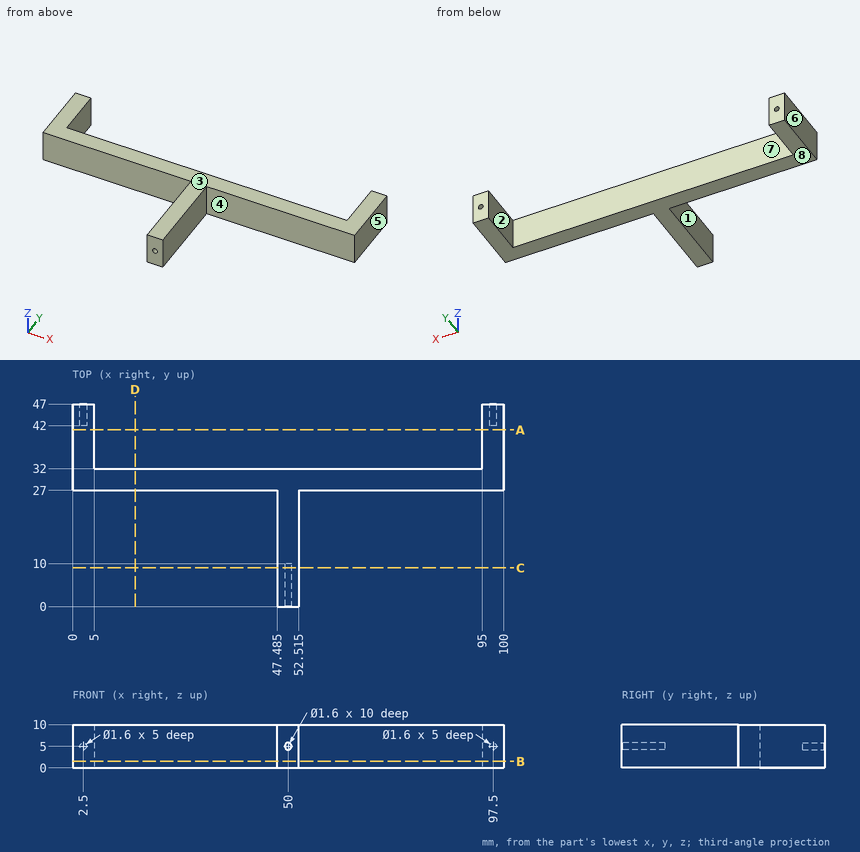
Check sheet for the drawn part. Datum: minimum x, y, z corner. Units: mm. A direction names the side the tool comes from. Give positions to 0.01 mm unless a question says otherwise; leave off trailing zeros. Write each loop counter-clockwise with the first axis right and the second up, starting at its lowest first coordinate (ties: lowest second). Pieces come first, ordered by that corner, then holes. Notation, with made-up numbers: M -34,26.25 L 25,26.25 A4 cw 25,32.25 Z; hole C 51,77.25 d3. An arc over 180 degrees is marked long. One line per question, with ' | ' between items.
1) Section check B-B on z = 1.5. Enter the section's corners in (x, y) (1 decimal), plus the area to 3 significant figures.
Result:
outline: M 0,27 L 47.5,27 L 47.5,0 L 52.5,0 L 52.5,27 L 100,27 L 100,47 L 95,47 L 95,32 L 5,32 L 5,47 L 0,47 Z | area: 786 mm2
2) Mould release check, pull along X, two halves, no side actions. Record for the marked faces 5, 6, 7 and 8: released by +X, released by -X, zero draft, split by the parting line, or undercut.
Result:
face 5: released by +X | face 6: released by -X | face 7: undercut | face 8: zero draft
3) Section check D-D on x = 14.5. Enter the section's corners in (y, z), plus the area to 3 significant figures.
Result:
outline: M 27,0 L 32,0 L 32,10 L 27,10 Z | area: 50.0 mm2
4) Gauge pin test, flat ends, axial feed: pin 1 Ø3 at (x, z) = (83, 4) entering from -Y; pin 2 Ø1 at (x, z) = (97.5, 5) entering from +Y; pin 3 Ø4 at (y, z) = (17.5, 7) entering from +X (1 decimal); pin 4 Ø3 at (y, z) = (42.5, 3) entering from -X. Record the tip position at first contact, or that the pin passes through.
Result:
pin 1: stops at y = 27 | pin 2: stops at y = 42 | pin 3: stops at x = 52.5 | pin 4: stops at x = 0
5) Section check A-A on y = 41. Enter the section's corners in (x, z), plus the area to 3 significant figures.
Result:
outline: M 0,0 L 5,0 L 5,10 L 0,10 Z; M 95,0 L 100,0 L 100,10 L 95,10 Z | area: 100 mm2
6) Section check C-C on y = 9. Enter the section's corners in (x, z) (1 decimal).
Result:
outline: M 47.5,0 L 52.5,0 L 52.5,10 L 47.5,10 Z; hole C 50,5 d1.6
7) Set-up check for the marked faces 1, 2, 3 and 4: record each of +Z, -Z, +X, -X, +Y, -Y from which the full face is reachable in a straight line by a thin tool's end or side.
Result:
face 1: +Z, -Z, -X, -Y | face 2: +Z, -Z, +Y | face 3: +Z, +X, -X, +Y, -Y | face 4: +Z, -Z, +X, -Y
8) Thickness scan on line 1 along X through (y, z) = (45.75, 5); line 2 along X through (y, z) = (38, 1); line 3 along Z through (x, y) = (50, 4.5). Record the ranges inside material, lowest first. Write a range as [from, to].
Result:
line 1: x = [0, 1.7], [3.3, 5], [95, 96.7], [98.3, 100] | line 2: x = [0, 5], [95, 100] | line 3: z = [0, 4.2], [5.8, 10]
